from build123d import *
from build123d.topology import SkipClean

# Parameters (mm, degrees)
SKETCH1_R           = 12
BOSS_EXTRUDE1_DEPTH = 3.175
BOSS_EXTRUDE2_START = 3.81
SKETCH2_R           = 12
BOSS_EXTRUDE2_DEPTH = 3.81
SKETCH3_R           = 3.937
CUT_EXTRUDE1_DEPTH  = 134.099089527
SKETCH4_R           = 1.27
CUT_EXTRUDE2_DEPTH  = 134.099089527
CUT_EXTRUDE3_DEPTH  = 133.970273023


with BuildPart() as part:
    # Sketch1 → Boss-Extrude1 (new body)
    with BuildSketch(Plane.XY):
        with BuildLine():
            ThreePointArc((79.156979953, 34.616777747), (78.764409425, 33.207913627), (78.648230314, 31.75))
            Line((78.648230314, 31.75), (93.886132052, 31.75))
            ThreePointArc((93.886132052, 31.75), (93.886918896, 31.813218964), (93.887181183, 31.876442281))
            ThreePointArc((93.887181183, 31.876442281), (87.66085737, 39.367908538), (79.156979953, 34.616777747))
        make_face()
        with BuildLine():
            ThreePointArc((87.4395, 24.347161532), (88.598049964, 24.621688616), (89.699693339, 25.073335615))
            ThreePointArc((89.699693339, 25.073335615), (92.723044454, 27.828451492), (93.886132052, 31.75))
            Line((93.886132052, 31.75), (78.648230314, 31.75))
            ThreePointArc((78.648230314, 31.75), (79.141141445, 29.177561465), (80.476005529, 26.924))
            Line((80.476005529, 26.924), (87.4395, 26.924))
            Line((87.4395, 26.924), (87.4395, 24.347161532))
        make_face()
        with BuildLine():
            Line((87.4395, 26.924), (80.476005529, 26.924))
            ThreePointArc((80.476005529, 26.924), (82.246043304, 25.403819152), (84.393093646, 24.490496444))
            ThreePointArc((84.393093646, 24.490496444), (85.909052633, 24.264862685), (87.4395, 24.347161532))
            Line((87.4395, 24.347161532), (87.4395, 26.924))
        make_face()
        with BuildLine():
            ThreePointArc((89.699693339, 25.073335615), (94.483227873, 27.711788353), (99.06, 30.694537484))
            Line((99.06, 30.694537484), (99.06, 31.75))
            Line((99.06, 31.75), (93.886132052, 31.75))
            ThreePointArc((93.886132052, 31.75), (92.723044454, 27.828451492), (89.699693339, 25.073335615))
        make_face()
        with BuildLine():
            ThreePointArc((99.06, 30.694537484), (106.888760949, 37.054762789), (113.784062988, 44.416608597))
            ThreePointArc((113.784062988, 44.416608597), (96.436063978, 43.110085278), (96.014300162, 60.502100346))
            ThreePointArc((96.014300162, 60.502100346), (86.225733854, 48.445051897), (79.156979953, 34.616777747))
            ThreePointArc((79.156979953, 34.616777747), (87.66085737, 39.367908538), (93.887181183, 31.876442281))
            ThreePointArc((93.887181183, 31.876442281), (93.886918896, 31.813218964), (93.886132052, 31.75))
            Line((93.886132052, 31.75), (99.06, 31.75))
            Line((99.06, 31.75), (99.06, 30.694537484))
        make_face()
        with Locations((104.48925, 52.0065)):
            Circle(SKETCH1_R)
    extrude(amount=BOSS_EXTRUDE1_DEPTH)

    # Sketch2 → Boss-Extrude2 (add)
    with SkipClean():  # the faces are left unmerged after this step: merging them gives an invalid solid
        with BuildSketch(Plane(origin=(0, 0, 0), x_dir=(-1, 0, 0), z_dir=(0, 0, -1)).offset(BOSS_EXTRUDE2_START)):
            with Locations((-104.48925, 52.0065)):
                Circle(SKETCH2_R)
        extrude(amount=-BOSS_EXTRUDE2_DEPTH)

    # Sketch3 → Cut-Extrude1 (cut, through all)
    with SkipClean():  # the faces are left unmerged after this step: merging them gives an invalid solid
        with BuildSketch(Plane(origin=(0, 0, -3.81), x_dir=(-1, 0, 0), z_dir=(0, 0, -1))):
            with Locations((-104.48925, 52.0065)):
                Circle(SKETCH3_R)
        extrude(amount=-CUT_EXTRUDE1_DEPTH, mode=Mode.SUBTRACT)

    # Sketch4 → Cut-Extrude2 (cut, through all)
    with SkipClean():  # the faces are left unmerged after this step: merging them gives an invalid solid
        with BuildSketch(Plane(origin=(0, 0, -3.81), x_dir=(-1, 0, 0), z_dir=(0, 0, -1))):
            with Locations((-112.99825, 52.0065)):
                Circle(SKETCH4_R)
            with Locations((-95.98025, 52.0065)):
                Circle(SKETCH4_R)
            with Locations((-104.48925, 60.5155)):
                Circle(SKETCH4_R)
            with Locations((-104.48925, 43.4975)):
                Circle(SKETCH4_R)
        extrude(amount=-CUT_EXTRUDE2_DEPTH, mode=Mode.SUBTRACT)

    # Sketch5 → Cut-Extrude3 (cut, through all)
    with SkipClean():  # the faces are left unmerged after this step: merging them gives an invalid solid
        with BuildSketch(Plane(origin=(0, 0, 0), x_dir=(-1, 0, 0), z_dir=(0, 0, -1))):
            with BuildLine():
                ThreePointArc((-104.430493989, 40.006643845), (-109.606684651, 41.15238269), (-113.7840634, 44.4166091))
                ThreePointArc((-113.7840634, 44.4166091), (-102.758092767, 33.479680706), (-89.699693406, 25.073335649))
                ThreePointArc((-89.699693406, 25.073335649), (-92.462895691, 27.440507008), (-93.81346398, 30.819079549))
                ThreePointArc((-93.81346398, 30.819079549), (-97.397477458, 37.40567327), (-104.430493989, 40.006643845))
            make_face()
        extrude(amount=-CUT_EXTRUDE3_DEPTH, mode=Mode.SUBTRACT)
    add(part.part.scale(1), mode=Mode.REPLACE)  # the faces are merged on a copy


solid = part.part
Input: part model. Units: mm. Frame: model coordinates. Give positions to 0.01 mm unless a question says otherwise; leave off trailing zeros. Order: outer loops, then holes, each group sorted by start corner. A loop starts at its lowest first (then second) coordinate and runs counter-clockwise, first axis right, second up.
Q1. Section B-B on y = 39.5. Output: boundary loops of the cut face in (x, z) (3 decimals), and give its area (3 significant figures).
Checked values:
outline: (81.242, 0) - (101.129, 0) - (101.129, 3.175) - (81.242, 3.175) - close
area: 63.1 mm2
Q2. Ray query, probe 1 along Y at (x, z) = (105, -3); probe 2 along X at (y, z) = (52.5, 2.5); probe 3 along Z at (x, y) = (82.5, 27) (3 decimals). Return the intervals inside material, ascending.
Checked values:
probe 1: y = 40.02 to 42.33, 44.66 to 48.1, 55.91 to 59.35, 61.68 to 64
probe 2: x = 89.06 to 94.81, 97.15 to 100.58, 108.4 to 111.83, 114.17 to 116.48
probe 3: z = 0 to 3.175
Q3. Section C-C on x = 110. Output: boundary loops of the cut face in (y, z) (3 decimals), and give its area (3 significant figures).
Checked values:
outline: (41.347, -3.81) - (62.666, -3.81) - (62.666, 3.175) - (41.347, 3.175) - close
area: 149 mm2
Q4. Contact query for flat-ended pins moving along their axis: pin 1 Ø1 at (x, z) = (111.5, 0) entering from +Y; pin 2 Ø8 at (x, y) = (87, 32) entering from -Z; pin 3 Ø2 at (y, z) = (53.5, 1) entering from +X. Output: stop coordinate, or through.
Checked values:
pin 1: stops at y = 62.09
pin 2: stops at z = 0
pin 3: stops at x = 116.48
Q5. Draft query along X for faces 1 (the cylindrical face through (86.345, 48.627, 1.565)), 2 (the cylindrical face through (104.655, 61.775, -0.366)), 3 (the flat face through (97, 44, 3.175)), 4 (the cylindrical face through (94.77, 52.39, -0.37)). Return one class per face: +X half, -X half, draft (parallel to the pull), parting line (faces both ways), or undercut.
Checked values:
face 1: -X half
face 2: undercut
face 3: draft
face 4: undercut
Q6. Section A-A on z = 0.75. Output: boundary loops of the cut face in (x, y).
Checked values:
outline: (79.16, 34.62) arc R7.62 ccw (long way) to (93.81, 30.82) arc R10.67 cw to (104.43, 40.01) arc R12 ccw (long way) to (96.01, 60.5) arc R74.31 ccw to start; hole circle Ø2.54 at (95.98, 52.01); hole circle Ø7.87 at (104.49, 52.01); hole circle Ø2.54 at (104.49, 43.5); hole circle Ø2.54 at (104.49, 60.52); hole circle Ø2.54 at (113, 52.01)
Q7. Section D-D on y = 58. Output: boundary loops of the cut face in (x, z) (3 decimals).
Checked values:
outline: (93.62, 0) - (94.093, 0) - (94.093, -3.81) - (114.885, -3.81) - (114.885, 3.175) - (93.62, 3.175) - close
